Can you work these out from the drawing? Everything is in mm from the part's minimum corner. Round coordinates to 2 decimals unless told otherwise and drop trailing zeros. Order: outer loops, then holes, each group sorted by start corner. A loop starts at its lowest first (then second) coordinate and runs counter-clockwise, first axis right, second up. Notation, with made-up numbers: (77, 15) -> (134, 15) arc R25 cw to (134, 44) -> close; hole circle Ø10 at (17.25, 21.5). An arc over 180 degrees is marked (long way). One line per item, written item: value.
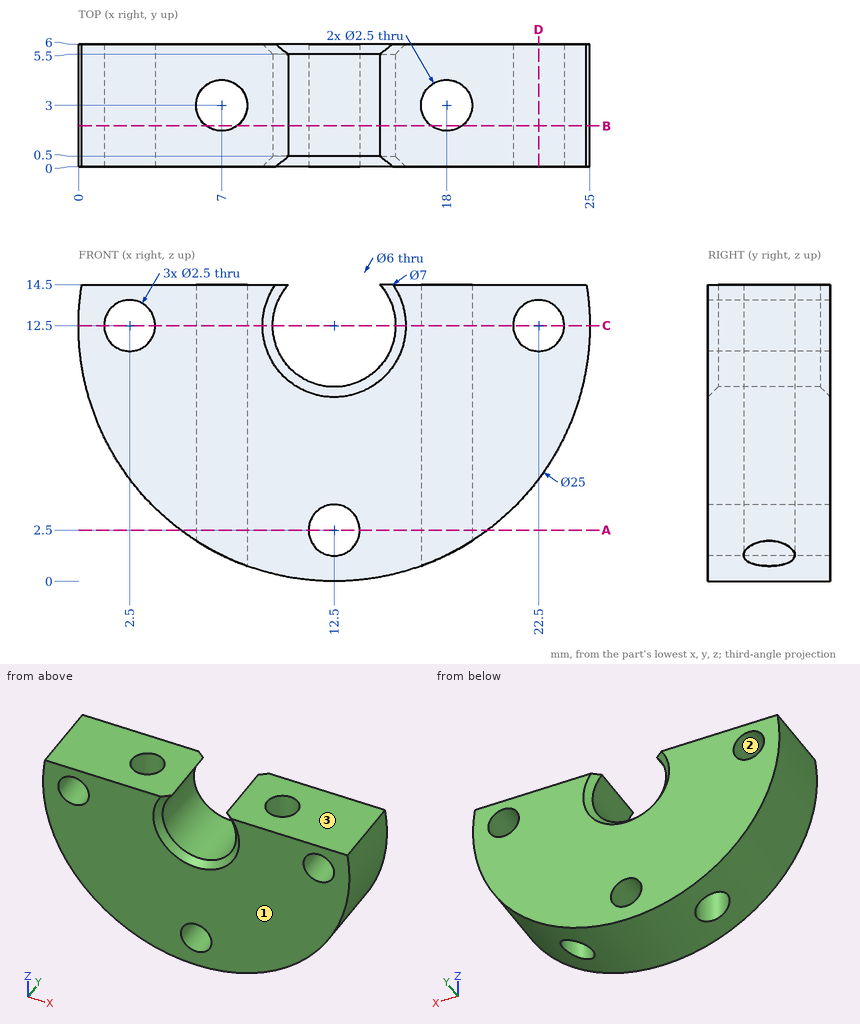
Q1. Will these pins go through, and if not, where does the flat tip stop? pin 1 Ø2 at (y, z) = (1, 5) entering from -X; pin 2 Ø3.5 at (x, z) = (12.5, 12.5) entering from +Y; pin 3 Ø4 at (x, z) = (12.5, 2.5) entering from -Y; pin 4 Ø3 at (x, z) = (12, 11) entering from +Y.
Answers below:
pin 1: x = 1.82
pin 2: through
pin 3: y = 0
pin 4: y = 5.58
Q2. I want a section at A-A on z = 2.5. List the corners of the cut face in (x, y) for me, plus the area to 3 significant figures.
Answers below:
outline: (5, 0) -> (11.25, 0) -> (11.25, 6) -> (5, 6) -> close; (13.75, 0) -> (20, 0) -> (20, 6) -> (13.75, 6) -> close; hole circle Ø2.5 at (7, 3); hole circle Ø2.5 at (18, 3)
area: 65.2 mm^2
Q3. Please list where these lines run through material, in increasing order: line 1 along X through (y, z) = (1, 12.75); line 2 along Y through (x, z) = (18, 10.25); line 3 along X through (y, z) = (5, 13.25).
Answers below:
line 1: 0 to 1.28, 3.72 to 9.51, 15.49 to 21.28, 23.72 to 25
line 2: 0 to 1.75, 4.25 to 6
line 3: 0.02 to 1.5, 3.5 to 9.6, 15.4 to 21.5, 23.5 to 24.98
Q4. I want a section at D-D on x = 22.5. List the corners of the cut face in (y, z) for me, plus the area to 3 significant figures.
Answers below:
outline: (0, 5) -> (6, 5) -> (6, 11.25) -> (0, 11.25) -> close; (0, 13.75) -> (6, 13.75) -> (6, 14.5) -> (0, 14.5) -> close
area: 42.0 mm^2
Q5. I want a section at C-C on z = 12.5. List the corners of the cut face in (x, y) for me, plus the area to 3 significant figures.
Answers below:
outline: (0, 0) -> (1.25, 0) -> (1.25, 6) -> (0, 6) -> close; (3.75, 0) -> (9, 0) -> (9.5, 0.5) -> (9.5, 5.5) -> (9, 6) -> (3.75, 6) -> close; (15.5, 0.5) -> (16, 0) -> (21.25, 0) -> (21.25, 6) -> (16, 6) -> (15.5, 5.5) -> close; (23.75, 0) -> (25, 0) -> (25, 6) -> (23.75, 6) -> close; hole circle Ø2.5 at (7, 3); hole circle Ø2.5 at (18, 3)
area: 73.7 mm^2
Q6. We'd pull the mould along Z, two halves only. Please class the marked faces 1, 2 and 3: released by +Z, released by -Z, zero draft, split by the parting line, or undercut.
Answers below:
face 1: zero draft
face 2: undercut
face 3: released by +Z
Q7. I want a section at B-B on y = 2. List the corners of the cut face in (x, z) for me, plus the area to 3 significant figures.
Answers below:
outline: (0.16, 14.5) arc R12.5 ccw to (6.25, 1.67) -> (6.25, 14.5) -> close; (7.75, 0.94) arc R12.5 ccw to (17.25, 0.94) -> (17.25, 14.5) -> (14.74, 14.5) arc R3 cw (long way) to (10.26, 14.5) -> (7.75, 14.5) -> close; (18.75, 1.67) arc R12.5 ccw to (24.84, 14.5) -> (18.75, 14.5) -> close; hole circle Ø2.5 at (2.5, 12.5); hole circle Ø2.5 at (12.5, 2.5); hole circle Ø2.5 at (22.5, 12.5)
area: 216 mm^2
